Geometry check sheet. Reference: the model listing, model coordinates, mm. A direction names the side the tool comes from. Coordinates: 2 decimals unless noted, no trailing zeros. Write each loop counter-clockwise with the first axis right and the second up, starting at its lowest first coordinate (ties: lowest second). Pieces come first, ordered by that corner, then holes. Notation, with made-up numbers: (38.25, -4.75) -> (85.25, -4.75) arc R34 cw to (85.25, 29.25) -> close; hole circle Ø10 at (-5, -3.5). An arc over 180 degrees is marked (long way). One line per question, with ' | ' between items.
```python
from build123d import *

# Parameters (mm, degrees)
SKETCH013_R     = 3.75
SKETCH013_R_2   = 1.75
SKETCH013_W     = 7
SKETCH013_H     = 7
PAD004_DEPTH    = 3
PAD_DEPTH       = 10
SKETCH015_R     = 1.75
POCKET005_DEPTH = 5
SKETCH004_R     = 1.75
POCKET006_DEPTH = 5
SKETCH014_R     = 1.75
POCKET007_DEPTH = 5
POCKET_DEPTH    = 2


with BuildPart() as part:
    # Sketch013 → Pad004 (new body)
    with BuildSketch(Plane.XY):
        Polygon((0, 65), (150, 65.000002), (150, -65), (0, -65), align=None)
        with Locations((13, 25)):
            Circle(SKETCH013_R, mode=Mode.SUBTRACT)
        with Locations((58, 25)):
            Circle(SKETCH013_R, mode=Mode.SUBTRACT)
        with Locations((13, -30)):
            Circle(SKETCH013_R, mode=Mode.SUBTRACT)
        with Locations((58, -30)):
            Circle(SKETCH013_R, mode=Mode.SUBTRACT)
        with Locations((146, 61.000002)):
            Circle(SKETCH013_R_2, mode=Mode.SUBTRACT)
        with Locations((146, -61)):
            Circle(SKETCH013_R_2, mode=Mode.SUBTRACT)
        with Locations((81.000022, 44.539576)):
            Circle(SKETCH013_R_2, mode=Mode.SUBTRACT)
        with Locations((136, 44.539576)):
            Circle(SKETCH013_R_2, mode=Mode.SUBTRACT)
        with Locations((80.901087, -45.46037)):
            Circle(SKETCH013_R_2, mode=Mode.SUBTRACT)
        with Locations((135.901066, -45.46037)):
            Circle(SKETCH013_R_2, mode=Mode.SUBTRACT)
        with Locations((90.500022, 44.539576)):
            Rectangle(SKETCH013_W, SKETCH013_H, mode=Mode.SUBTRACT)
        with Locations((108.500011, 44.519789)):
            Rectangle(SKETCH013_W, SKETCH013_H, mode=Mode.SUBTRACT)
        with Locations((126.5, 44.500002)):
            Rectangle(SKETCH013_W, SKETCH013_H, mode=Mode.SUBTRACT)
        with Locations((90.480235, 26.539587)):
            Rectangle(SKETCH013_W, SKETCH013_H, mode=Mode.SUBTRACT)
        with Locations((108.480224, 26.5198)):
            Rectangle(SKETCH013_W, SKETCH013_H, mode=Mode.SUBTRACT)
        with Locations((126.480213, 26.500013)):
            Rectangle(SKETCH013_W, SKETCH013_H, mode=Mode.SUBTRACT)
        with Locations((90.460448, 8.539598)):
            Rectangle(SKETCH013_W, SKETCH013_H, mode=Mode.SUBTRACT)
        with Locations((108.460437, 8.519811)):
            Rectangle(SKETCH013_W, SKETCH013_H, mode=Mode.SUBTRACT)
        with Locations((126.460426, 8.500024)):
            Rectangle(SKETCH013_W, SKETCH013_H, mode=Mode.SUBTRACT)
        with Locations((90.440661, -9.460392)):
            Rectangle(SKETCH013_W, SKETCH013_H, mode=Mode.SUBTRACT)
        with Locations((108.44065, -9.480178)):
            Rectangle(SKETCH013_W, SKETCH013_H, mode=Mode.SUBTRACT)
        with Locations((126.440639, -9.499965)):
            Rectangle(SKETCH013_W, SKETCH013_H, mode=Mode.SUBTRACT)
        with Locations((90.420874, -27.460381)):
            Rectangle(SKETCH013_W, SKETCH013_H, mode=Mode.SUBTRACT)
        with Locations((108.420863, -27.480168)):
            Rectangle(SKETCH013_W, SKETCH013_H, mode=Mode.SUBTRACT)
        with Locations((126.420852, -27.499954)):
            Rectangle(SKETCH013_W, SKETCH013_H, mode=Mode.SUBTRACT)
        with Locations((90.401087, -45.46037)):
            Rectangle(SKETCH013_W, SKETCH013_H, mode=Mode.SUBTRACT)
        with Locations((108.401076, -45.480157)):
            Rectangle(SKETCH013_W, SKETCH013_H, mode=Mode.SUBTRACT)
        with Locations((126.401066, -45.499944)):
            Rectangle(SKETCH013_W, SKETCH013_H, mode=Mode.SUBTRACT)
    extrude(amount=PAD004_DEPTH)

    # Sketch001 (on DatumPlane) → Pad (join)
    with BuildSketch(Plane.XY.offset(3)):
        Polygon((0, 55), (3, 55), (128, 55), (128, 52), (3, 52), (3, -62), (128, -62), (128, -65), (3, -65), (0, -65), align=None)
    extrude(amount=PAD_DEPTH)

    # Sketch015 → Pocket005 (cut)
    with BuildSketch(Plane.XZ.offset(65)):
        with Locations((25, 9.5)):
            Circle(SKETCH015_R)
        with Locations((75, 9.5)):
            Circle(SKETCH015_R)
        with Locations((125, 9.5)):
            Circle(SKETCH015_R)
    extrude(amount=-POCKET005_DEPTH, mode=Mode.SUBTRACT)

    # Sketch004 (on DatumPlane) → Pocket006 (cut, symmetric)
    with BuildSketch(Plane.XZ.offset(-55)):
        with Locations((25, 9.5)):
            Circle(SKETCH004_R)
        with Locations((75, 9.5)):
            Circle(SKETCH004_R)
        with Locations((125, 9.5)):
            Circle(SKETCH004_R)
    extrude(amount=POCKET006_DEPTH, both=True, mode=Mode.SUBTRACT)

    # Sketch014 → Pocket007 (cut)
    with BuildSketch(Plane.YZ):
        with Locations((45, 9.5)):
            Circle(SKETCH014_R)
        with Locations((-5, 9.5)):
            Circle(SKETCH014_R)
        with Locations((-55, 9.5)):
            Circle(SKETCH014_R)
    extrude(amount=POCKET007_DEPTH, mode=Mode.SUBTRACT)

    # Sketch → Pocket (cut)
    with BuildSketch(Plane.XY.offset(3.5)):
        Polygon((83.55, 52), (134.15, 52), (134.15, 42.5), (140, 42.5), (140, -42.5), (134.15, -42.5), (134.15, -53), (83.55, -53), (83.55, -42.5), (72.55, -42.5), (72.55, 42.5), (83.55, 42.5), align=None)
    extrude(amount=-POCKET_DEPTH, mode=Mode.SUBTRACT)


solid = part.part
```
(1) Depth check by flat-ended pin: P1, Ø4, axis at x = 48.5, z = 5.5, coming from the +Y side; P2, Ø1.5, axis at x = 50, y = 50, coming from the +Z side. Enter the tip coordinate at first touch or a pass-through.
Answers below:
P1: stops at y = 55 | P2: stops at z = 3
(2) Draft check along Z on faces 4 (the face through (2.7, -4.7, 13)), 5 (the face through (137.669, 45.065, 1.479)), 6 (the face through (1.479, -5.228, 11.235)). Enter one of: pulls with the +Z half, pulls with the -Z half, needs draft (parallel to the pull), parting line crosses it, or undercut.
Answers below:
face 4: pulls with the +Z half | face 5: needs draft | face 6: undercut
(3) Material ranges on line 1 (Y direction, x = 58, z = 2.2); line 2 (Y direction, x = 75, z = 6.75); line 3 (X direction, y = 37, z = 1.75), recorded low to high.
Answers below:
line 1: y = -65 to -33.75, -26.25 to 21.25, 28.75 to 65 | line 2: y = -65 to -62, 52 to 55 | line 3: x = 0 to 72.55, 140 to 150
(4) Cross-section at A-A (x = 75). Record the cut outline in (y, z).
Answers below:
outline: (-65, 0) -> (65, 0) -> (65, 3) -> (55, 3) -> (55, 7.75) -> (52, 7.75) -> (52, 3) -> (42.5, 3) -> (42.5, 1.5) -> (-42.5, 1.5) -> (-42.5, 3) -> (-62, 3) -> (-62, 7.75) -> (-65, 7.75) -> close; (-65, 11.25) -> (-62, 11.25) -> (-62, 13) -> (-65, 13) -> close; (52, 11.25) -> (55, 11.25) -> (55, 13) -> (52, 13) -> close
(5) Tool access check on faces 1 (the face through (59, 1, 3)), 2 (the face through (65, 55, 8)), 3 (the face through (76.669, -63.521, 10.026)). Record the directions out of +Z, -Z, +X, -X, +Y, -Y that give a thin tool (end or side, any length) a straight path to the whole face; none if there is none.
Answers below:
face 1: +Z, +X | face 2: +Z, +X, -X, +Y | face 3: +Y, -Y
(6) Cross-section at D-D (x = 102). Record the cut outline in (y, z).
Answers below:
outline: (-65, 0) -> (65, 0) -> (65, 3) -> (55, 3) -> (55, 13) -> (52, 13) -> (52, 1.5) -> (-53, 1.5) -> (-53, 3) -> (-62, 3) -> (-62, 13) -> (-65, 13) -> close
(7) Cross-section at C-C (y = -55). Record the cut outline in (x, z), plus the area to 4 significant figures.
Answers below:
outline: (0, 0) -> (150, 0) -> (150, 3) -> (3, 3) -> (3, 7.75) -> (0, 7.75) -> close; (0, 11.25) -> (3, 11.25) -> (3, 13) -> (0, 13) -> close | area: 469.5 mm²
(8) Cross-section at B-B (y = -10.5). Record the cut outline in (x, z).
Answers below:
outline: (0, 0) -> (86.94, 0) -> (86.94, 1.5) -> (72.55, 1.5) -> (72.55, 3) -> (3, 3) -> (3, 13) -> (0, 13) -> close; (93.94, 0) -> (104.94, 0) -> (104.94, 1.5) -> (93.94, 1.5) -> close; (111.94, 0) -> (122.94, 0) -> (122.94, 1.5) -> (111.94, 1.5) -> close; (129.94, 0) -> (150, 0) -> (150, 3) -> (140, 3) -> (140, 1.5) -> (129.94, 1.5) -> close
